```python
from build123d import *

# Parameters (mm, degrees)
CIRCLE001_R      = 1.937531
EXTRUDE011_DEPTH = 10
EXTRUDE001_W     = 39.873674
EXTRUDE001_H     = 10
EXTRUDE004_DEPTH = 10


with BuildPart() as extrude011:
    # Circle001 → Extrude011 (new body)
    with BuildSketch(Plane(origin=(10.504012, -11.75601, 0), x_dir=(1, 0, 0), z_dir=(0, 0, 1))):
        Circle(CIRCLE001_R)
    extrude(amount=EXTRUDE011_DEPTH)


with BuildPart() as cut001:
    # Extrude001 → Extrude004 (new body)
    with BuildSketch(Plane(origin=(12.214123, 2.775603, 5), x_dir=(-0.612281, -0.790641, 0), z_dir=(0.790641, -0.612281, 0))):
        Rectangle(EXTRUDE001_W, EXTRUDE001_H)
    extrude(amount=EXTRUDE004_DEPTH)

    # Cut001: cut Extrude011
    add(extrude011.part, mode=Mode.SUBTRACT)


solid = cut001.part
```
Geometry: final body of the model. Coordinates: model frame, mm. Coordinates: 2 decimals unless noted, no trailing zeros. Loops run counter-clockwise (first coordinate to the right, second up) from the corner with the lowest first, then second, coordinate; pieces in that order, holes last. Notation, with made-up numbers: M -32.75,-40 L 1.25,-40 A9 cw 1.25,-29 Z; hole C -17.75,12 d11. An arc over 180 degrees is marked long. Put each result on its own line as item: value.
(1) Cut plane D-D on x = 25. Return the cut outline in (y, z).
Answer sheet:
outline: M 2.95,0 L 18.09,0 L 18.09,10 L 2.95,10 Z
(2) Draft query along Y for faces 1 (the face through (16, 0, 10)), 2 (the face through (11.546, -10.122, 4.93)), 3 (the face through (28.32, 15.52, 5.07)). Return one class per face: pulls with the +Y half, pulls with the -Y half, needs draft (parallel to the pull), parting line crosses it, or undercut.
Answer sheet:
face 1: needs draft
face 2: undercut
face 3: pulls with the +Y half
(3) Cut plane C-C on y = 10.5. Return the cut outline in (x, z), then the cut area to 3 significant figures.
Answer sheet:
outline: M 18.2,0 L 30.84,0 L 30.84,10 L 18.2,10 Z
area: 126 mm^2
(4) Cut plane A-A on x = 9. Return the cut outline in (y, z), then the cut area to 3 significant figures.
Answer sheet:
outline: M -17.71,0 L -12.98,0 L -12.98,10 L -17.71,10 Z; M -10.53,0 L -1.37,0 L -1.37,10 L -10.53,10 Z
area: 139 mm^2
(5) First-contact query: pin 1 (3 mm diameter, centred on y = -1, z = 4, fed in from -X); pin 2 (2 mm diameter, centred on x = 12.5, y = 3.5, fed in from +Z); pin 3 (6 mm diameter, centred on y = -8.5, z = 7.5, fed in from -X); pin 4 (6 mm diameter, centred on x = 15, z = 8.5, fed in from -Y). Flat tips, straight axial feed; report the tip coordinate or a pass-through.
Answer sheet:
pin 1: stops at x = 8.13
pin 2: stops at z = 10
pin 3: stops at x = 1.16
pin 4: stops at y = -13.83
(6) Material intervals for probe 1 along X at (y, z) = (-10, 3); probe 2 along X at (y, z) = (-13.5, 3.75); probe 3 along Y at (x, z) = (11, 7.5), sorted ascending.
Answer sheet:
probe 1: x = 2.32 to 9.69, 11.32 to 14.97
probe 2: x = 0.67 to 9.66, 11.35 to 12.26
probe 3: y = -15.12 to -13.63, -9.88 to 1.21
(7) Cut plane B-B on z = 1.5. Return the cut outline in (x, y), then the cut area to 3 significant figures.
Answer sheet:
outline: M 0.01,-12.99 L 7.91,-19.11 L 32.33,12.42 L 24.42,18.54 Z; hole C 10.5,-11.76 d3.88
area: 387 mm^2
